```python
from build123d import *

# Parameters (mm, degrees)
F0_R     = 2.4765
F0_R_2   = 8.001
F1_DEPTH = 2.9718


with BuildPart() as f1:
    # F0 (on Front) → F1 (new body)
    with BuildSketch(Plane.XZ):
        with BuildLine():
            Line((-19.05, 0), (-19.05, -203.2))
            ThreePointArc((-19.05, -203.2), (0, -222.25), (19.05, -203.2))
            Line((19.05, -203.2), (19.05, 0))
            ThreePointArc((19.05, 0), (0, 19.05), (-19.05, 0))
        make_face()
        with Locations((-10.795, -190.5)):
            Circle(F0_R, mode=Mode.SUBTRACT)
        with Locations((0, -203.2)):
            Circle(F0_R_2, mode=Mode.SUBTRACT)
        with Locations((10.795, -190.5)):
            Circle(F0_R, mode=Mode.SUBTRACT)
        with BuildLine():
            ThreePointArc((7.9375, -177.8), (0, -185.7375), (-7.9375, -177.8))
            Line((-7.9375, -177.8), (-7.9375, -6.35))
            ThreePointArc((-7.9375, -6.35), (0, 1.5875), (7.9375, -6.35))
            Line((7.9375, -6.35), (7.9375, -177.8))
        make_face(mode=Mode.SUBTRACT)
        with Locations((0, 12.7)):
            Circle(F0_R, mode=Mode.SUBTRACT)
    extrude(amount=F1_DEPTH)


solid = f1.part
```
Can you work these out from the model? Positions are in its coordinate system, mm. A direction names the side the tool comes from. Coordinates: 2 decimals unless noted, no trailing zeros. Order: outer loops, then holes, each group sorted by start corner. A loop starts at its lowest first (then second) coordinate and runs counter-clockwise, first axis right, second up.
1. If we section it at A-A (x = 0): Please give me the cut outline in (y, z).
2. I'm going to push a flat-ended pin straight in: pin 1 (3 mm diameter, centred on x = 0, z = 12.7, fed in from -Y). Where does the tip first touch, or does it pass through?
3. Thinking about a two-plate mould opening in Z: for faces 1 (the face through (-0.419, -1.465, -222.245)), 2 (the face through (-11.117, -1.465, -188.045)), 3 (the face through (-0.537, -1.465, 10.282)), 4 (the face through (8.2, -2.972, -99.9)), which applies, +Z half, -Z half, draft (parallel to the pull), parting line (faces both ways), or undercut?
4. If we section it at C-C (y = -0.95): Give the number of separate pieces and of enclosed holes in the cut face, then the cut area to 3 significant figures.
5. If we section it at B-B (z = -11.5): Please give me the cut outline in (x, y).
6. If we section it at D-D (z = 12.7): Please give me the cut outline in (x, y), then the cut area to 3 significant figures.
7. For faces 5 (the face through (0.175, -1.465, -185.736)), 6 (the face through (0.419, -1.465, 19.045)), which set-ups out of +Z, -Z, +X, -X, +Y, -Y let a thin tool reach every point of the face, with its end or its side?
8. I need wall thicknesses on line 1 (Z direction, x = 0, y = -1.25); line 2 (X direction, y = -1.55, z = -190.5); line 3 (X direction, y = -0.45, z = -62.5). Which ranges of each line are inside material? Lowest first, please.
Entries:
1. outline: (-2.97, -222.25) - (0, -222.25) - (0, -211.2) - (-2.97, -211.2) - close; (-2.97, -195.2) - (0, -195.2) - (0, -185.74) - (-2.97, -185.74) - close; (-2.97, 1.59) - (0, 1.59) - (0, 10.22) - (-2.97, 10.22) - close; (-2.97, 15.18) - (0, 15.18) - (0, 19.05) - (-2.97, 19.05) - close
2. pin 1: passes through
3. face 1: -Z half
3. face 2: undercut
3. face 3: undercut
3. face 4: draft
4. separate pieces: 1
4. enclosed holes: 5
4. area: 5,700 mm2
5. outline: (-19.05, -2.97) - (-7.94, -2.97) - (-7.94, 0) - (-19.05, 0) - close; (7.94, -2.97) - (19.05, -2.97) - (19.05, 0) - (7.94, 0) - close
6. outline: (-14.2, -2.97) - (-2.48, -2.97) - (-2.48, 0) - (-14.2, 0) - close; (2.48, -2.97) - (14.2, -2.97) - (14.2, 0) - (2.48, 0) - close
6. area: 69.7 mm2
7. face 5: +Y, -Y
7. face 6: +Z, +Y, -Y
8. line 1: z = -222.25 to -211.2, -195.2 to -185.74, 1.59 to 10.22, 15.18 to 19.05
8. line 2: x = -19.05 to -13.27, -8.32 to 8.32, 13.27 to 19.05
8. line 3: x = -19.05 to -7.94, 7.94 to 19.05
